Job drawing, mm, ordinate dimensions from the low corner. One solid piece. A direction names the side the tool comes from. Give positions to 0.01 mm unless a question says otherwise; leave off trailing zeros. Order: outer loops, then holes, each group sorted by start corner. A loop starts at its lowest first (then second) coordinate and runs counter-clockwise, first axis right, second up.
Item 1: Band-saw the part on A-A on z = 10.5. Give the cut face in (x, y).
Item 2: Flat gauge pins, fed straight in: P1, Ø2, axis at x = 115.5, y = 36, coming from the -Z side; P2, Ø10, axis at x = 154.5, y = 54, coming from the -Z side; P3, Ø4, axis at x = 35, y = 38.5, coming from the -Z side. Where does each tip first touch, or does it go through?
Item 3: Wall check: L1, parallel to X at y = 33, z = 4; L2, parallel to X at y = 45, z = 47.5; L3, parallel to Z at x = 47, y = 55. Give the ranges that are in metal, low to high.
Item 4: Band-saw the part on B-B on y = 60.5. Give the cut face in (x, z), plus the area to 3 significant figures.
Item 5: Band-saw the part on D-D on x = 41. Give the cut face in (y, z), plus the area to 3 significant figures.
Item 6: Which spindle directions (+Z, -Z, +X, -X, +Y, -Y) get a long thin tool onto all of the face, cutting with end or side? Do the marked faces 5 and 6. Say none if no direction does.
Item 7: Two-plate mould, pull along X, no slides. Class the marked faces 1, 2, 3 and 4: released by +X, released by -X, zero draft, split by the parting line, or undercut.
Item 8: Band-saw the part on C-C on x = 110.5. Give the cut face in (y, z).
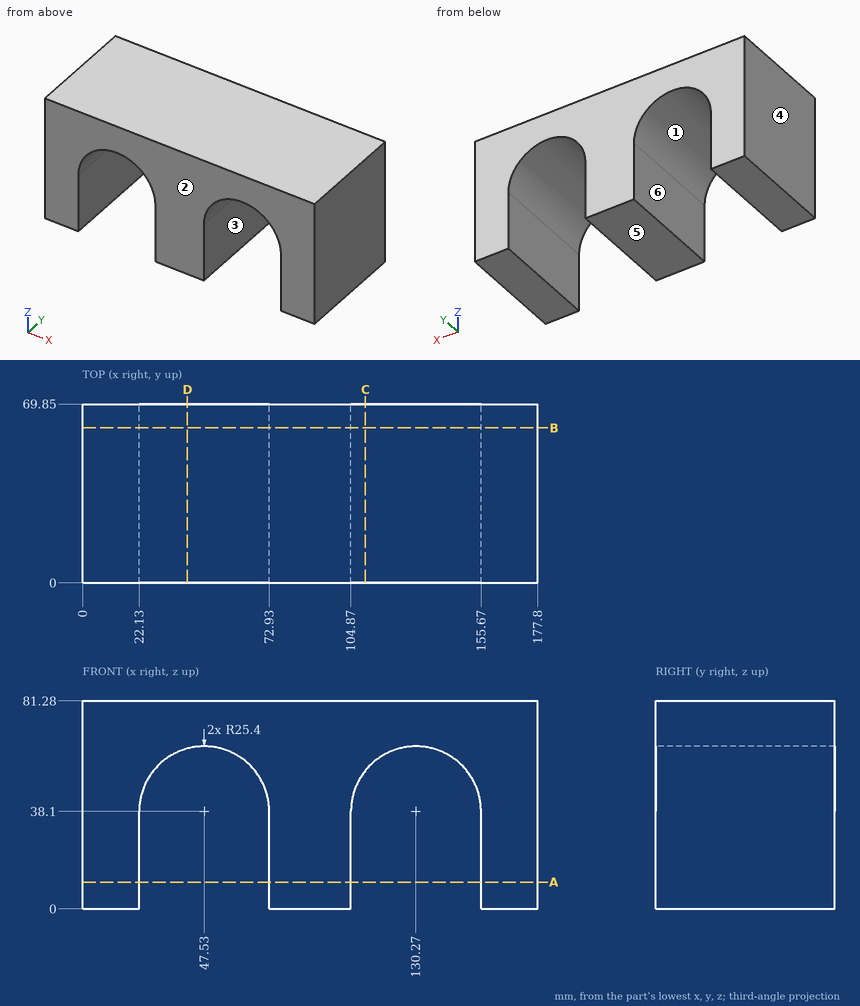
The answers:
1. outline: (0, 0) - (22.13, 0) - (22.13, 69.85) - (0, 69.85) - close; (72.93, 0) - (104.87, 0) - (104.87, 69.85) - (72.93, 69.85) - close; (155.67, 0) - (177.8, 0) - (177.8, 69.85) - (155.67, 69.85) - close
2. P1: stops at z = 58.01
2. P2: stops at z = 0
2. P3: stops at z = 58.93
3. L1: x = 0 to 22.13, 72.93 to 104.87, 155.67 to 177.8
3. L2: x = 0 to 23.93, 71.13 to 106.67, 153.87 to 177.8
3. L3: z = 63.49 to 81.28
4. outline: (0, 0) - (22.13, 0) - (22.13, 38.1) arc R25.4 cw to (72.93, 38.1) - (72.93, 0) - (104.87, 0) - (104.87, 38.1) arc R25.4 cw to (155.67, 38.1) - (155.67, 0) - (177.8, 0) - (177.8, 81.28) - (0, 81.28) - close
4. area: 8,550 mm2
5. outline: (0, 62.65) - (69.85, 62.65) - (69.85, 81.28) - (0, 81.28) - close
5. area: 1,300 mm2
6. face 5: -Z, +X, -X, +Y, -Y
6. face 6: -Z, +Y, -Y
7. face 1: undercut
7. face 2: zero draft
7. face 3: undercut
7. face 4: released by -X
8. outline: (0, 54.05) - (69.85, 54.05) - (69.85, 81.28) - (0, 81.28) - close
